```python
from build123d import *

# Parameters (mm, degrees)
SKETCH1_W           = 101.6
SKETCH1_H           = 101.6
BOSS_EXTRUDE1_DEPTH = 12.7
SKETCH4_W           = 47.2
SKETCH4_H           = 47.2
BOSS_EXTRUDE3_DEPTH = 23
SKETCH5_W           = 42.3
SKETCH5_H           = 42.3
CUT_EXTRUDE1_DEPTH  = 32
SKETCH6_R           = 11
SKETCH6_R_2         = 1.5
SKETCH6_R_3         = 1.715206785
SKETCH6_R_4         = 1.661518809
CUT_EXTRUDE2_DEPTH  = 10
SKETCH7_W           = 5.3
SKETCH7_H           = 10
CUT_EXTRUDE3_DEPTH  = 5
SKETCH8_W           = 5.3
SKETCH8_H           = 10
CUT_EXTRUDE5_DEPTH  = 12.7
SKETCH9_R           = 6.35
CUT_EXTRUDE6_DEPTH  = 12.7


with BuildPart() as part:
    # Sketch1 → Boss-Extrude1 (new body)
    with BuildSketch(Plane.XY):
        with Locations((50.8, 50.8)):
            Rectangle(SKETCH1_W, SKETCH1_H)
    extrude(amount=BOSS_EXTRUDE1_DEPTH)

    # Sketch4 → Boss-Extrude3 (add)
    with BuildSketch(Plane.XY.offset(12.7)):
        with Locations((50.8, 50.8)):
            Rectangle(SKETCH4_W, SKETCH4_H)
    extrude(amount=BOSS_EXTRUDE3_DEPTH)

    # Sketch5 → Cut-Extrude1 (cut)
    with BuildSketch(Plane(origin=(0, 0, 0), x_dir=(-1, 0, 0), z_dir=(0, 0, -1))):
        with Locations((-50.45, 50.45)):
            Rectangle(SKETCH5_W, SKETCH5_H)
    extrude(amount=-CUT_EXTRUDE1_DEPTH, mode=Mode.SUBTRACT)

    # Sketch6 → Cut-Extrude2 (cut)
    with BuildSketch(Plane.XY.offset(35.7)):
        with Locations((50.8, 50.8)):
            Circle(SKETCH6_R)
        with Locations((35.3, 66.3)):
            Circle(SKETCH6_R_2)
        with Locations((66.3, 66.3)):
            Circle(SKETCH6_R_3)
        with Locations((66.3, 35.3)):
            Circle(SKETCH6_R_4)
        with Locations((35.3, 35.3)):
            Circle(SKETCH6_R_2)
    extrude(amount=-CUT_EXTRUDE2_DEPTH, mode=Mode.SUBTRACT)

    # Sketch7 → Cut-Extrude3 (cut)
    with BuildSketch(Plane.ZY.offset(-27.2)):
        with Locations((15.35, 50.8)):
            Rectangle(SKETCH7_W, SKETCH7_H)
    extrude(amount=-CUT_EXTRUDE3_DEPTH, mode=Mode.SUBTRACT)

    # Sketch8 → Cut-Extrude5 (cut)
    with BuildSketch(Plane.XY.offset(12.7)):
        with Locations((24.55, 50.8)):
            Rectangle(SKETCH8_W, SKETCH8_H)
    extrude(amount=-CUT_EXTRUDE5_DEPTH, mode=Mode.SUBTRACT)

    # Sketch9 → Cut-Extrude6 (cut)
    with BuildSketch(Plane(origin=(0, 0, 0), x_dir=(-1, 0, 0), z_dir=(0, 0, -1))):
        with Locations((-88.9, 88.9)):
            Circle(SKETCH9_R)
        with Locations((-12.7, 88.9)):
            Circle(SKETCH9_R)
        with Locations((-12.7, 12.7)):
            Circle(SKETCH9_R)
        with Locations((-88.9, 12.7)):
            Circle(SKETCH9_R)
    extrude(amount=-CUT_EXTRUDE6_DEPTH, mode=Mode.SUBTRACT)


solid = part.part
```
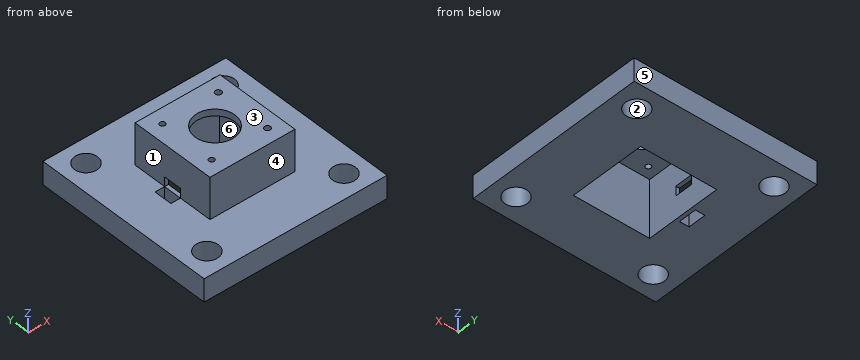
Geometry: final body of the model. Coordinates: model frame, mm. Face numbers are marked on the shaded views. A direction names the side the tool comes from. Round coordinates to 2 decimals unless told otherwise and drop trailing zeros. Order: outer loops, then holes, each group sorted by start corner. A loop starts at its lowest first (then second) coordinate and runs counter-clockwise, first axis right, second up. Notation, with made-up numbers: (-3.75, 69.25) -> (14.25, 69.25) arc R14 ccw to (14.25, 87.25) -> close; hole circle Ø2 at (57, 27). An arc over 180 degrees is marked (long way). Use one line per item in the form item = value.
(1) Access query for the marked faces 4, 5 and 6. Directions: +Z, -Z, +X, -X, +Y, -Y. A direction counts if a zero-diameter tool reaches every point of the face in a straight line with its end or side. Return the directions, or none.
Results list:
face_4 = +Z, +X, -X, -Y
face_5 = +Z, -Z, +X, -X, +Y
face_6 = -Z
(2) Section D-D on z = 19.5. Return loops of the section in (x, y).
Results list:
outline = (27.2, 27.2) -> (74.4, 27.2) -> (74.4, 74.4) -> (27.2, 74.4) -> close; hole (29.3, 29.3) -> (71.6, 29.3) -> (71.6, 71.6) -> (29.3, 71.6) -> close
(3) Section C-C on x = 88.9. Return loops of the section in (y, z), and give its area (3 significant figures).
Results list:
outline = (0, 0) -> (6.35, 0) -> (6.35, 12.7) -> (0, 12.7) -> close; (19.05, 0) -> (82.55, 0) -> (82.55, 12.7) -> (19.05, 12.7) -> close; (95.25, 0) -> (101.6, 0) -> (101.6, 12.7) -> (95.25, 12.7) -> close
area = 968 mm^2
(4) Section A-A on x = 25. Return loops of the section in (y, z), and give its area (3 significant figures).
Results list:
outline = (0, 0) -> (45.8, 0) -> (45.8, 12.7) -> (0, 12.7) -> close; (55.8, 0) -> (101.6, 0) -> (101.6, 12.7) -> (55.8, 12.7) -> close
area = 1,160 mm^2
(5) Section B-B on y = 66.3. Return loops of the section in (x, z), and give its area (3 significant figures).
Results list:
outline = (0, 0) -> (29.3, 0) -> (29.3, 32) -> (33.8, 32) -> (33.8, 35.7) -> (27.2, 35.7) -> (27.2, 12.7) -> (0, 12.7) -> close; (36.8, 32) -> (64.58, 32) -> (64.58, 35.7) -> (36.8, 35.7) -> close; (68.02, 32) -> (71.6, 32) -> (71.6, 0) -> (101.6, 0) -> (101.6, 12.7) -> (74.4, 12.7) -> (74.4, 35.7) -> (68.02, 35.7) -> close
area = 999 mm^2
(6) First-contact query: pin 1 Ø2 at (y, z) = (43.5, 27.5) entering from -X; pin 2 Ø1 at (x, y) = (59, 65.5) entering from -Z; pin 3 Ø4 at (x, y) = (19.5, 73) entering from +Z. Flat tips, straight axial feed; report the tip coordinate or a pass-through.
Results list:
pin_1 = 27.2
pin_2 = 32
pin_3 = 12.7
(7) Ray query, probe 1 along X at (y, z) = (13, 9); probe 2 along X at (y, z) = (46.5, 6.5); probe 3 along Y at (x, z) = (66.3, 34.85). Return the intervals inside material, ascending. Write a range as [from, to].
Results list:
probe_1 = [0, 6.36], [19.04, 82.56], [95.24, 101.6]
probe_2 = [0, 21.9], [27.2, 29.3], [71.6, 101.6]
probe_3 = [27.2, 33.64], [36.96, 64.58], [68.02, 74.4]
(8) Draft query along X for the marked faces 1, 2 and 3. Return one class per face: pulls with the +X half, pulls with the -X half, needs draft (parallel to the pull), parting line crosses it, or undercut.
Results list:
face_1 = pulls with the -X half
face_2 = undercut
face_3 = needs draft
